```python
from build123d import *

# Parameters (mm, degrees)
CROQUIS1_W              = 35
CROQUIS1_H              = 35
CROQUIS1_R              = 1.25
CROQUIS1_R_2            = 6.5
SALIENTE_EXTRUIR1_DEPTH = 5
CORTAR_EXTRUIR1_DEPTH   = 2
CHAFL_N1_SIZE           = 1.25


with BuildPart() as part:
    # Croquis1 → Saliente-Extruir1 (new body)
    with BuildSketch(Plane.XY):
        Rectangle(CROQUIS1_W, CROQUIS1_H)
        with Locations((-15.37, 15.37)):
            Circle(CROQUIS1_R, mode=Mode.SUBTRACT)
        with Locations((15.37, 15.37)):
            Circle(CROQUIS1_R, mode=Mode.SUBTRACT)
        with Locations((15.37, -15.37)):
            Circle(CROQUIS1_R, mode=Mode.SUBTRACT)
        with Locations((-15.37, -15.37)):
            Circle(CROQUIS1_R, mode=Mode.SUBTRACT)
        Circle(CROQUIS1_R_2, mode=Mode.SUBTRACT)
        with Locations((13.3, 0)):
            Circle(CROQUIS1_R, mode=Mode.SUBTRACT)
        with Locations((-13.3, 0)):
            Circle(CROQUIS1_R, mode=Mode.SUBTRACT)
    extrude(amount=SALIENTE_EXTRUIR1_DEPTH)

    # Croquis2 → Cortar-Extruir1 (cut)
    with BuildSketch(Plane.XY.offset(5)):
        Polygon((-13.3, 3.464101615), (-16.3, 1.732050808), (-16.3, -1.732050808), (-13.3, -3.464101615), (-10.3, -1.732050808), (-10.3, 1.732050808), align=None)
        Polygon((13.3, 3.464101615), (10.3, 1.732050808), (10.3, -1.732050808), (13.3, -3.464101615), (16.3, -1.732050808), (16.3, 1.732050808), align=None)
    extrude(amount=-CORTAR_EXTRUIR1_DEPTH, mode=Mode.SUBTRACT)

    # Chaflán1
    # the kernel refuses this chamfer: 1.25 mm, written as the material it takes off along each edge
    with BuildSketch(Plane(origin=(-15.37, 15.37, 0), x_dir=(1, 0, 0), z_dir=(0, -1, 0))) as chafl_n1_piece_1:
        Polygon((1.25 + CHAFL_N1_SIZE, 0), (1.25, CHAFL_N1_SIZE), (1.25, 0), align=None)
    revolve(axis=Axis((-15.37, 15.37, 0), (0, 0, 1)), mode=Mode.SUBTRACT)
    with BuildSketch(Plane(origin=(15.37, 15.37, 0), x_dir=(1, 0, 0), z_dir=(0, -1, 0))) as chafl_n1_piece_2:
        Polygon((1.25 + CHAFL_N1_SIZE, 0), (1.25, CHAFL_N1_SIZE), (1.25, 0), align=None)
    revolve(axis=Axis((15.37, 15.37, 0), (0, 0, 1)), mode=Mode.SUBTRACT)
    with BuildSketch(Plane(origin=(15.37, -15.37, 0), x_dir=(1, 0, 0), z_dir=(0, -1, 0))) as chafl_n1_piece_3:
        Polygon((1.25 + CHAFL_N1_SIZE, 0), (1.25, CHAFL_N1_SIZE), (1.25, 0), align=None)
    revolve(axis=Axis((15.37, -15.37, 0), (0, 0, 1)), mode=Mode.SUBTRACT)
    with BuildSketch(Plane(origin=(-15.37, -15.37, 0), x_dir=(1, 0, 0), z_dir=(0, -1, 0))) as chafl_n1_piece_4:
        Polygon((1.25 + CHAFL_N1_SIZE, 0), (1.25, CHAFL_N1_SIZE), (1.25, 0), align=None)
    revolve(axis=Axis((-15.37, -15.37, 0), (0, 0, 1)), mode=Mode.SUBTRACT)


solid = part.part
```
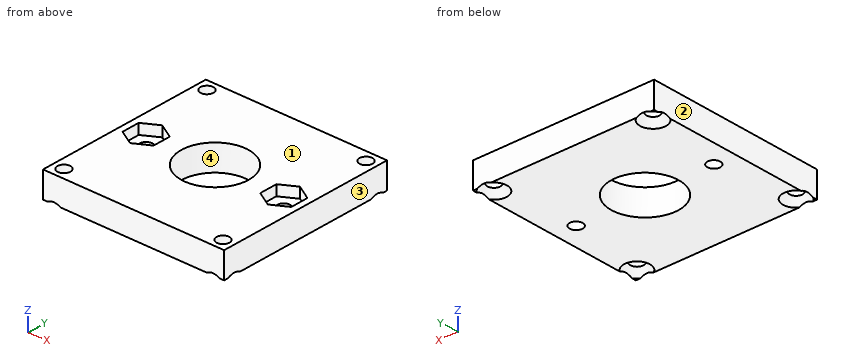
The listing builds one solid part. Answer for the finished solid, in the listing's coordinates (mm). Face numbers are marked on the shaded views. Round coordinates to 2 decimals unless told otherwise and drop trailing zeros. Loops run counter-clockwise (first coordinate to the right, second up) from the corner with the lowest first, then second, coordinate; pieces in that order, holes last. Notation, with made-up numbers: (77, 18.5) - (94, 18.5) arc R23 ccw to (94, 28.5) - close; hole circle Ø3 at (64, -28.5). An arc over 180 degrees is marked (long way). Use one line per item in the form item = value. Start each with the question number.
1. Consider line 1 (Y direction, x = -13.3, z = 2.3); line 2 (X direction, y = -0.5, z = 2.25); line 3 (Y direction, x = 0, z = 1.25). Determine where each line is inside the solid, lowest interval first. Write a range as [from, to].
2. The part is cut by section A-A on x = 0. Determine the outline of the cut face in (y, z).
3. For a pull along X with two mould halves and no side action, classify the marked faces 1, 2, 3 and 4 as pulls with the +X half, pulls with the -X half, needs draft (parallel to the pull), parting line crosses it, or undercut.
4. The part is cut by section C-C on y = 0. Determine the outline of the cut face in (x, z), then the cut area to 3 significant figures.
5. Given pin 1 Ø3 at (x, y) = (13.3, 0) entering from +Z, flat-ended and moving along its own axis, determine where the tip first touches the part or whether it passes through.
6. The part is cut by section B-B on y = 15.37. Determine the outline of the cut face in (x, z).
7. The part is cut by section D-D on z = 3.4. Determine the outline of the cut face in (x, y), then the cut area to 3 significant figures.
Geometry check:
q1.line_1 = [-17.5, -1.25], [1.25, 17.5]
q1.line_2 = [-17.5, -14.45], [-12.15, -6.48], [6.48, 12.15], [14.45, 17.5]
q1.line_3 = [-17.5, -6.5], [6.5, 17.5]
q2.outline = (-17.5, 0) - (-6.5, 0) - (-6.5, 5) - (-17.5, 5) - close; (6.5, 0) - (17.5, 0) - (17.5, 5) - (6.5, 5) - close
q3.face_1 = needs draft
q3.face_2 = pulls with the -X half
q3.face_3 = pulls with the +X half
q3.face_4 = undercut
q4.outline = (-17.5, 0) - (-14.55, 0) - (-14.55, 3) - (-16.3, 3) - (-16.3, 5) - (-17.5, 5) - close; (-12.05, 0) - (-6.5, 0) - (-6.5, 5) - (-10.3, 5) - (-10.3, 3) - (-12.05, 3) - close; (6.5, 0) - (12.05, 0) - (12.05, 3) - (10.3, 3) - (10.3, 5) - (6.5, 5) - close; (14.55, 0) - (17.5, 0) - (17.5, 5) - (16.3, 5) - (16.3, 3) - (14.55, 3) - close
q4.area = 71.0 mm^2
q5.pin_1 = 3
q6.outline = (-17.5, 0.37) - (-16.62, 1.25) - (-16.62, 5) - (-17.5, 5) - close; (-14.12, 1.25) - (-12.87, 0) - (12.87, 0) - (14.12, 1.25) - (14.12, 5) - (-14.12, 5) - close; (16.62, 1.25) - (17.5, 0.37) - (17.5, 5) - (16.62, 5) - close
q7.outline = (-17.5, -17.5) - (17.5, -17.5) - (17.5, 17.5) - (-17.5, 17.5) - close; hole circle Ø2.5 at (-15.37, -15.37); hole circle Ø2.5 at (-15.37, 15.37); hole (-16.3, -1.73) - (-13.3, -3.46) - (-10.3, -1.73) - (-10.3, 1.73) - (-13.3, 3.46) - (-16.3, 1.73) - close; hole circle Ø13 at (0, 0); hole (10.3, -1.73) - (13.3, -3.46) - (16.3, -1.73) - (16.3, 1.73) - (13.3, 3.46) - (10.3, 1.73) - close; hole circle Ø2.5 at (15.37, -15.37); hole circle Ø2.5 at (15.37, 15.37)
q7.area = 1,010 mm^2
